The listing builds one solid part. Answer for the finished solid, in the listing's coordinates (mm). A direction names the side the tool comes from. Coordinates: 2 decimals unless noted, no trailing zeros. Write each loop counter-clockwise with the first axis right and the second up, starting at its lowest first coordinate (ties: lowest second). Pieces come first, ordered by that corner, then holes. Notation, with made-up numbers: M -40,67 L 7,67 A23 ccw 7,93 Z; hole C 47.25,74 d11. An arc over 180 degrees is marked long. Answer as a JSON object with one key per item and string values. Group by question number.
from build123d import *

# Parameters (mm, degrees)
CYLINDER_R        = 1.5
CYLINDER_DEPTH    = 20
ARRAY_X_COUNT     = 2
ARRAY_X_PITCH     = 16
ARRAY_Y_COUNT     = 2
ARRAY_Y_PITCH     = 34
CYLINDER001_R     = 1.8
CYLINDER001_DEPTH = 10
BOX005_W          = 2
BOX005_H          = 3
BOX005_DEPTH      = 41
FILLET_R          = 1.5
BOX004_W          = 10
BOX004_H          = 9.6
BOX004_DEPTH      = 4
FILLET001_R       = 2
BOX001_W          = 17.4
BOX001_H          = 2
BOX001_DEPTH      = 41
BOX_W             = 41.4
BOX_H             = 42
BOX_DEPTH         = 3
BOX003_W          = 4
BOX003_H          = 31
BOX003_DEPTH      = 31
BOX002_W          = 4
BOX002_H          = 42
BOX002_DEPTH      = 41
BOX007_W          = 2
BOX007_H          = 22
BOX007_DEPTH      = 22
BOX006_W          = 2
BOX006_H          = 42
BOX006_DEPTH      = 41
CYLINDER002_R     = 2.5
CYLINDER002_DEPTH = 5
ARRAY001_X_COUNT  = 2
ARRAY001_X_PITCH  = 16
ARRAY001_Y_COUNT  = 2
ARRAY001_Y_PITCH  = 34


with BuildPart() as obj1:
    # Cylinder → Cylinder (new body)
    with BuildSketch(Plane(origin=(-23, 4, 0), x_dir=(1, 0, 0), z_dir=(0, 0, 1))):
        Circle(CYLINDER_R)
    extrude(amount=CYLINDER_DEPTH)

    # Array X: obj1_2


with BuildPart() as obj1_1:
    add(obj1.part)
    with Locations(*[(i * ARRAY_X_PITCH, 0, 0) for i in range(1, ARRAY_X_COUNT)]):
        add(obj1.part)

    # Array Y: obj1_2


with BuildPart() as obj1_2:
    add(obj1_1.part)
    with Locations(*[(0, i * ARRAY_Y_PITCH, 0) for i in range(1, ARRAY_Y_COUNT)]):
        add(obj1_1.part)


with BuildPart() as bolt_hole:
    # Cylinder001 → Cylinder001 (new body)
    with BuildSketch(Plane(origin=(5, -4, -3), x_dir=(1, 0, 0), z_dir=(0, 0, 1))):
        Circle(CYLINDER001_R)
    extrude(amount=CYLINDER001_DEPTH)


with BuildPart() as side_locker_fillet:
    # Box005 → Box005 (new body)
    with BuildSketch(Plane.XY):
        with Locations((1, 1.5)):
            Rectangle(BOX005_W, BOX005_H)
    extrude(amount=BOX005_DEPTH)

    # Fillet
    fillet_edges = [side_locker_fillet.edges().sort_by_distance(p)[0] for p in [
        (2, 3, 20.5),
    ]]
    fillet(fillet_edges, radius=FILLET_R)


with BuildPart() as bolt_hole_cube_fillet:
    # Box004 → Box004 (new body)
    with BuildSketch(Plane(origin=(0, -9.6, 0), x_dir=(1, 0, 0), z_dir=(0, 0, 1))):
        with Locations((5, 4.8)):
            Rectangle(BOX004_W, BOX004_H)
    extrude(amount=BOX004_DEPTH)

    # Fillet001
    fillet001_edges = [bolt_hole_cube_fillet.edges().sort_by_distance(p)[0] for p in [
        (0, -9.6, 2),
        (10, -9.6, 2),
    ]]
    fillet(fillet001_edges, radius=FILLET001_R)


with BuildPart() as side_cut:
    # Box001 → Box001 (new body)
    with BuildSketch(Plane.XY):
        with Locations((8.7, 1)):
            Rectangle(BOX001_W, BOX001_H)
    extrude(amount=BOX001_DEPTH)

    # Fusion: union side locker fillet, bolt hole cube fillet
    add(side_locker_fillet.part)
    add(bolt_hole_cube_fillet.part)

    # Cut001: cut bolt hole
    add(bolt_hole.part, mode=Mode.SUBTRACT)


with BuildPart() as bottom_cube:
    # Box → Box (new body)
    with BuildSketch(Plane(origin=(-26, 0, 0), x_dir=(1, 0, 0), z_dir=(0, 0, 1))):
        with Locations((20.7, 21)):
            Rectangle(BOX_W, BOX_H)
    extrude(amount=BOX_DEPTH)


with BuildPart() as part_mirroring:
    # Part__Mirroring: instance of side cut
    add(side_cut.part.mirror(Plane(origin=(0, 21, 0), x_dir=(1, 0, 0), z_dir=(0, 1, 0))))


with BuildPart() as light_wall_hole_cube:
    # Box003 → Box003 (new body)
    with BuildSketch(Plane(origin=(8, 5.5, 6.5), x_dir=(1, 0, 0), z_dir=(0, 0, 1))):
        with Locations((2, 15.5)):
            Rectangle(BOX003_W, BOX003_H)
    extrude(amount=BOX003_DEPTH)


with BuildPart() as light_wall:
    # Box002 → Box002 (new body)
    with BuildSketch(Plane(origin=(8, 0, 0), x_dir=(1, 0, 0), z_dir=(0, 0, 1))):
        with Locations((2, 21)):
            Rectangle(BOX002_W, BOX002_H)
    extrude(amount=BOX002_DEPTH)

    # Cut: cut light wall hole cube
    add(light_wall_hole_cube.part, mode=Mode.SUBTRACT)


with BuildPart() as filter_wall_hole_cube:
    # Box007 → Box007 (new body)
    with BuildSketch(Plane(origin=(8, 10, 11), x_dir=(1, 0, 0), z_dir=(0, 0, 1))):
        with Locations((1, 11)):
            Rectangle(BOX007_W, BOX007_H)
    extrude(amount=BOX007_DEPTH)


with BuildPart() as filter_wall:
    # Box006 → Box006 (new body)
    with BuildSketch(Plane(origin=(8, 0, 0), x_dir=(1, 0, 0), z_dir=(0, 0, 1))):
        with Locations((1, 21)):
            Rectangle(BOX006_W, BOX006_H)
    extrude(amount=BOX006_DEPTH)

    # Cut003: cut filter wall hole cube
    add(filter_wall_hole_cube.part, mode=Mode.SUBTRACT)


with BuildPart() as filter_wall_1:
    # Cut003 placement: moved
    add(filter_wall.part.moved(Location((7.4, 0, 0))))


with BuildPart() as lighter_holder_cut:
    # Cylinder002 → Cylinder002 (new body)
    with BuildSketch(Plane(origin=(-23, 4, 0), x_dir=(1, 0, 0), z_dir=(0, 0, 1))):
        Circle(CYLINDER002_R)
    extrude(amount=CYLINDER002_DEPTH)

    # Array001 X: lighter holder cut ×2


with BuildPart() as lighter_holder_cut_1:
    add(lighter_holder_cut.part)
    with Locations(*[(i * ARRAY001_X_PITCH, 0, 0) for i in range(1, ARRAY001_X_COUNT)]):
        add(lighter_holder_cut.part)

    # Array001 Y: lighter holder cut ×2


with BuildPart() as lighter_holder_cut_2:
    add(lighter_holder_cut_1.part)
    with Locations(*[(0, i * ARRAY001_Y_PITCH, 0) for i in range(1, ARRAY001_Y_COUNT)]):
        add(lighter_holder_cut_1.part)

    # Fusion001: union side cut, bottom cube, Part__Mirroring, light wall, filter wall
    add(side_cut.part)
    add(bottom_cube.part)
    add(part_mirroring.part)
    add(light_wall.part)
    add(filter_wall_1.part)

    # Cut002: cut obj1
    add(obj1_2.part, mode=Mode.SUBTRACT)


solid = lighter_holder_cut_2.part
Item 1: A cutting plane is placed at A-A, the plane y = 23. Write down the section's boundary in (x, z).
Item 2: A tool of negligible diameter and unlimited length cuts with its end or side. For faces 4 (the face through (10, 36.5, 22)), 5 (the face through (-5.66, 6.11, 3.99)), 6 (the face through (16, 21, 11)), from which of +Z, -Z, +X, -X, +Y, -Y can it reach the whole face along a straight path? Write none if from no direction.
Item 3: A cutting plane is placed at C-C, the plane z = 19. Write down the section's boundary in (x, y), and give its area (3 significant figures).
Item 4: Consider L1, parallel to Y at x = -7, z = 2; L2, parallel to Y at x = 5, z = 1; L3, parallel to X at y = 4, z = 2. Determine where each line is inside the solid, lowest interval first. Write a range as from..to.
Item 5: For a pull along Z with two mould halves and no side action, classify faces 1 (the face through (-7, 2, 5)), 2 (the face through (10, 5.5, 22)), 3 (the face through (5, 51.6, 2)) as +Z half, -Z half, draft (parallel to the pull), parting line (faces both ways), or undercut.
Item 6: A cutting plane is placed at B-B, the plane x = -7. Write down the section's boundary in (y, z), and give its area (3 significant figures).
Item 7: Flat-ended cylindrical pins translate along their axes: pin 1 Ø4 at (x, y) = (-7, 4) entering from -Z; pin 2 Ø2.5 at (x, z) = (-12, 2) entering from -Y; pin 3 Ø7.5 at (x, y) = (6.5, 48.5) entering from +Z; pin 4 Ø4 at (y, z) = (-0.5, 15) entering from -X. Find the tip coordinate at first contact, or state that the pin passes through.
Item 8: A cutting plane is placed at D-D, the plane y = 46. Write down the section's boundary in (x, z), and give its area (3 significant figures).
Answer:
{
 "1": {"outline": "M -26,0 L 17.4,0 L 17.4,11 L 15.4,11 L 15.4,3 L 12,3 L 12,6.5 L 8,6.5 L 8,3 L -26,3 Z; M 8,37.5 L 12,37.5 L 12,41 L 8,41 Z; M 15.4,33 L 17.4,33 L 17.4,41 L 15.4,41 Z"},
 "2": {"face 4": "-X", "face 5": "+Z", "face 6": "+X, -X"},
 "3": {"outline": "M 0,0 L 17.4,0 L 17.4,10 L 15.4,10 L 15.4,2 L 12,2 L 12,5.5 L 8,5.5 L 8,2 L 1.91,2 A1.5 ccw 0.5,3 L 0,3 Z; M 0,39 L 0.5,39 A1.5 ccw 1.91,40 L 8,40 L 8,36.5 L 12,36.5 L 12,40 L 15.4,40 L 15.4,32 L 17.4,32 L 17.4,42 L 0,42 Z", "area": "133 mm2"},
 "4": {"L1": "0..2.5, 5.5..36.5, 39.5..42", "L2": "-9.6..-5.8, -2.2..44.2, 47.8..51.6", "L3": "-26..-24.5, -21.5..-8.5, -5.5..17.4"},
 "5": {"face 1": "+Z half", "face 2": "undercut", "face 3": "draft"},
 "6": {"outline": "M 0,0 L 2.5,0 L 2.5,5 L 1.5,5 L 1.5,3 L 0,3 Z; M 5.5,0 L 36.5,0 L 36.5,5 L 35.5,5 L 35.5,3 L 6.5,3 L 6.5,5 L 5.5,5 Z; M 39.5,0 L 42,0 L 42,3 L 40.5,3 L 40.5,5 L 39.5,5 Z", "area": "116 mm2"},
 "7": {"pin 1": "z = 0", "pin 2": "y = 0", "pin 3": "z = 4", "pin 4": "x = 0"},
 "8": {"outline": "M 0,0 L 3.2,0 L 3.2,4 L 0,4 Z; M 6.8,0 L 10,0 L 10,4 L 6.8,4 Z", "area": "25.6 mm2"}
}
